Here's how the part is built. I have some questions about the finished solid (model axes, mm). A direction names the side the tool comes from. Round coordinates to 2 decimals unless told otherwise and drop trailing zeros. Loops run counter-clockwise (first coordinate to the right, second up) from the corner with the lowest first, then second, coordinate; pieces in that order, holes last. Notation, with made-up numbers: M 86,34 L 109,34 A14 cw 109,49 Z; hole C 27,82.5 d9. An arc over 180 degrees is marked long. Use a Markdown table: item, result.
from build123d import *

# Parameters (mm, degrees)
EXTRUDE_1_DEPTH     = 50
CUT_EXTRUDE_1_DEPTH = 10
CUT_EXTRUDE_2_DEPTH = 10
EXTRUDE_2_DEPTH     = 15


with BuildPart() as part:
    # 草图1 → 凸台-拉伸1 (new body)
    with BuildSketch(Plane.XY):
        with BuildLine():
            Line((4, 0), (20, 0))
            Line((20, 0), (20, 20))
            Line((20, 20), (0, 20))
            Line((0, 20), (0, 4))
            ThreePointArc((0, 4), (1.171572875, 1.171572875), (4, 0))
        make_face()
    extrude(amount=EXTRUDE_1_DEPTH)

    # 草图2 → 切除-拉伸1 (cut)
    with BuildSketch(Plane.ZY):
        with BuildLine():
            Line((3, 15.5), (13, 15.5))
            ThreePointArc((13, 15.5), (15.65, 12.85), (13, 10.2))
            Line((13, 10.2), (3, 10.2))
            ThreePointArc((3, 10.2), (0.35, 12.85), (3, 15.5))
        make_face()
        with BuildLine():
            Line((23, 15.5), (33, 15.5))
            ThreePointArc((33, 15.5), (35.65, 12.85), (33, 10.2))
            Line((33, 10.2), (23, 10.2))
            ThreePointArc((23, 10.2), (20.35, 12.85), (23, 15.5))
        make_face()
        with BuildLine():
            Line((41, 15.5), (46, 15.5))
            ThreePointArc((46, 15.5), (48.65, 12.85), (46, 10.2))
            Line((46, 10.2), (41, 10.2))
            ThreePointArc((41, 10.2), (38.35, 12.85), (41, 15.5))
        make_face()
    extrude(amount=-CUT_EXTRUDE_1_DEPTH, mode=Mode.SUBTRACT)

    # 草图3 → 切除-拉伸2 (cut)
    with BuildSketch(Plane.XZ):
        with BuildLine():
            Line((15.5, 46), (15.5, 29))
            ThreePointArc((15.5, 29), (12.85, 26.35), (10.2, 29))
            Line((10.2, 29), (10.2, 46))
            ThreePointArc((10.2, 46), (12.85, 48.65), (15.5, 46))
        make_face()
        with BuildLine():
            Line((15.5, 20), (15.5, 5))
            ThreePointArc((15.5, 5), (12.85, 2.35), (10.2, 5))
            Line((10.2, 5), (10.2, 20))
            ThreePointArc((10.2, 20), (12.85, 22.65), (15.5, 20))
        make_face()
    extrude(amount=-CUT_EXTRUDE_2_DEPTH, mode=Mode.SUBTRACT)

    # 草图4 → 凸台-拉伸2 (add)
    with BuildSketch(Plane.XZ):
        Polygon((95, 42), (95, 50), (20, 50), (20, 42), (65, 42), (65, 8), (20, 8), (20, 0), (95, 0), (95, 8), (75, 8), (75, 42), align=None)
    extrude(amount=-EXTRUDE_2_DEPTH)


solid = part.part
1. For pin 1 Ø8 at (y, z) = (3, 41.5) entering from +X; pin 2 Ø3 at (y, z) = (18, 36) entering from +X; pin 3 Ø2.5 at (y, z) = (13.5, 31) entering from -X; pin 4 Ø8 at (x, z) = (84.5, 36) entering from +Y, each with a flat end and sliding along its axis, tell me the tip position at first contact or that it passes through.
Answer sheet:
| item | result |
|---|---|
| pin 1 | x = 95 |
| pin 2 | x = 20 |
| pin 3 | x = 10 |
| pin 4 | through |
2. Imagine slicing it at A-A, the plane z = 25. Write out the boundary of the cut face in (x, y).
Answer sheet:
| item | result |
|---|---|
| outline | M 0,4 A4 ccw 4,0 L 20,0 L 20,20 L 0,20 L 0,15.5 L 10,15.5 L 10,10.2 L 0,10.2 Z; M 65,0 L 75,0 L 75,15 L 65,15 Z |
3. Imagine slicing it at D-D, the plane y = 5.5. Write out the boundary of the cut face in (x, z).
Answer sheet:
| item | result |
|---|---|
| outline | M 0,0 L 95,0 L 95,8 L 75,8 L 75,42 L 95,42 L 95,50 L 0,50 Z; hole M 10.2,5 A2.65 ccw 15.5,5 L 15.5,20 A2.65 ccw 10.2,20 Z; hole M 10.2,29 A2.65 ccw 15.5,29 L 15.5,46 A2.65 ccw 10.2,46 Z; hole M 20,8 L 65,8 L 65,42 L 20,42 Z |
4. I need wall thicknesses on probe 1 along X at (y, z) = (6.25, 17); probe 2 along Z at (x, y) = (82, 7); probe 3 along X at (y, z) = (12.75, 29). Which ranges of each line are inside material? Lowest first, please. Write a range as from..to.
Answer sheet:
| item | result |
|---|---|
| probe 1 | 0..10.2, 15.5..20, 65..75 |
| probe 2 | 0..8, 42..50 |
| probe 3 | 10..20, 65..75 |
5. We'd pull the mould along X, two halves only. Please class faces 1 (the face through (65, 7, 25)), 2 (the face through (5, 10.2, 8)), 3 (the face through (95, 7, 46)): +X half, -X half, draft (parallel to the pull), parting line (faces both ways), or undercut.
Answer sheet:
| item | result |
|---|---|
| face 1 | undercut |
| face 2 | draft |
| face 3 | +X half |
6. Imagine slicing it at B-B, the plane x = 32. Write out the boundary of the cut face in (y, z), then the cut area to 3 significant figures.
Answer sheet:
| item | result |
|---|---|
| outline | M 0,0 L 15,0 L 15,8 L 0,8 Z; M 0,42 L 15,42 L 15,50 L 0,50 Z |
| area | 240 mm2 |
7. Imagine slicing it at C-C, the plane y = 12.85. Write out the boundary of the cut face in (x, z), then the cut area to 3 significant figures.
Answer sheet:
| item | result |
|---|---|
| outline | M 0,0 L 95,0 L 95,8 L 75,8 L 75,42 L 95,42 L 95,50 L 0,50 L 0,48.65 L 10,48.65 L 10,38.35 L 0,38.35 L 0,35.65 L 10,35.65 L 10,20.35 L 0,20.35 L 0,15.65 L 10,15.65 L 10,0.35 L 0,0.35 Z; hole M 20,8 L 65,8 L 65,42 L 20,42 Z |
| area | 2,130 mm2 |
8. Which directions (+Z, -Z, +X, -X, +Y, -Y) give clear straight access to the entire face, cutting with the end or side of a thin tool? Please do faces 4 (the face through (65.3, 15, 30.9)), 5 (the face through (43, 7, 8)), 6 (the face through (4.93, 12.79, 38.35)).
Answer sheet:
| item | result |
|---|---|
| face 4 | +Z, -Z, +X, +Y |
| face 5 | +Y, -Y |
| face 6 | -X |
